```python
from build123d import *

# Parameters (mm, degrees)
F0_W     = 76.2
F0_H     = 63.5
F1_DEPTH = 25.4
F2_W     = 18.529646
F2_H     = 29.221089
F3_DEPTH = 63.5
F4_W     = 18.529646
F4_H     = 14.610544
F5_DEPTH = 12.7


with BuildPart() as f1:
    # F0 (on Top) → F1 (new body)
    with BuildSketch(Plane.XY):
        with Locations((1.98446, 2.628666)):
            Rectangle(F0_W, F0_H)
    extrude(amount=F1_DEPTH)

    # F2 (on face) → F3 (join)
    with BuildSketch(Plane.XZ.offset(29.121334)):
        with Locations((-26.850717, 40.010544)):
            Rectangle(F2_W, F2_H)
    extrude(amount=-F3_DEPTH)

    # F4 (on face) → F5 (cut)
    with BuildSketch(Plane.XZ.offset(29.121334)):
        with Locations((-26.850717, 47.315817)):
            Rectangle(F4_W, F4_H)
    extrude(amount=-F5_DEPTH, mode=Mode.SUBTRACT)


solid = f1.part
```
Input: part model. Units: mm. Frame: model coordinates. A direction names the side the tool comes from. Give positions to 0.01 mm unless a question says otherwise; leave off trailing zeros. Loops run counter-clockwise (first coordinate to the right, second up) from the corner with the lowest first, then second, coordinate; pieces in that order, holes last.
1) Section query B-B on z = 48.5. Return the cut outline in (x, y).
A:
outline: (-36.12, -16.42) - (-17.59, -16.42) - (-17.59, 34.38) - (-36.12, 34.38) - close
2) Section query A-A on y = 3. Return the cut outline in (x, z).
A:
outline: (-36.12, 0) - (40.08, 0) - (40.08, 25.4) - (-17.59, 25.4) - (-17.59, 54.62) - (-36.12, 54.62) - close
3) Reachability of faces 1 (the flat face through (-27, -16.421, 47)), 2 (the flat face through (1, -29.121, 15)), 3 (the flat face through (-17.586, 2, 40)) from +Z, -Z, +X, -X, +Y, -Y: full face, straight path, thin tool, end or side. Return the list, or none.
A:
face 1: +Z, +X, -X, -Y
face 2: +Z, -Z, +X, -X, -Y
face 3: +Z, +X, +Y, -Y
4) Contact query for flat-ended pins moving along their axis: pin 1 (12 mm diameter, centred on x = -13, z = 46.5, fed in from -Y); pin 2 (23.5 mm diameter, centred on y = 5.5, z = 45, fed in from +X). Output: stop coordinate, or through.
A:
pin 1: stops at y = -16.42
pin 2: stops at x = -17.59
5) Section query D-D on y = -18. Return the cut outline in (x, z), and give its area (3 significant figures).
A:
outline: (-36.12, 0) - (40.08, 0) - (40.08, 25.4) - (-17.59, 25.4) - (-17.59, 40.01) - (-36.12, 40.01) - close
area: 2,210 mm2
6) Line query: L1, parallel to Z at x = 25, y = 12.5; L2, parallel to X at y = 17, z = 36; L3, parallel to Y at x = -29.5, z = 47. Output: solid intervals per line, ascending.
A:
L1: z = 0 to 25.4
L2: x = -36.12 to -17.59
L3: y = -16.42 to 34.38
7) Section query C-C on x = 1.5. Return the cut outline in (y, z).
A:
outline: (-29.12, 0) - (34.38, 0) - (34.38, 25.4) - (-29.12, 25.4) - close
